Here's how the part is built. I have some questions about the finished solid (model axes, mm). Round coordinates to 2 decimals unless told otherwise and drop trailing zeros. Order: outer loops, then holes, each group sorted by start corner. A loop starts at its lowest first (then second) coordinate and runs counter-clockwise, first axis right, second up.
Autodesk Inventor part; units mm, degrees
ref_plane "YZ Plane" through (0, 0, 0) normal (1, 0, 0) x (0, 1, 0)
ref_plane "XZ Plane" through (0, 0, 0) normal (0, 1, 0) x (-1, 0, 0)
ref_plane "XY Plane" through (0, 0, 0) normal (0, 0, 1) x (1, 0, 0)
sketch "Sketch14" plane through (0, 0, 0) normal (0, 0, 1) x (1, 0, 0)
  circle A0 centre (0, 0) radius 65
  dimension "d67" = 130
extrude "Extrusion10" add sketch "Sketch14" along normal blind 6
sketch "Sketch15" plane through (0, 0, 6) normal (0, 0, 1) x (1, 0, 0)
  circle A0 centre (-37.7323, 38.6299) radius 2
  line L0 (-37.7323, 38.6299) -> (0, 0) construction
  circle A1 centre (0, 0) radius 65
  line L1 (0, 0) -> (-55.3564, 56.6733) construction
  line L2 (-55.3564, 56.6733) -> (-63.1164, 49.0935) construction
  dimension "d70" = 54
  dimension "d75" = 4
extrude "Extrusion11" cut sketch "Sketch15" against normal blind 6 contours A0
sketch "Sketch16" plane through (0, 0, 6) normal (0, 0, 1) x (1, 0, 0)
  circle A0 centre (-37.7323, 38.6299) radius 2.75
  circle A1 centre (-37.7323, 38.6299) radius 2
  point P0 (0, 0)
  dimension "d73" = 5.5
extrude "Extrusion12" add sketch "Sketch16" along normal blind 8
sketch "Sketch17" plane through (0, 0, 6) normal (0, 0, 1) x (1, 0, 0)
  circle A0 centre (-37.7323, 38.6299) radius 2.75
  circle A1 centre (-37.7323, 38.6299) radius 2 construction
  line L0 (-37.7323, 38.6299) -> (0, 0) construction
  line L1 (-37.7323, 38.6299) -> (-45.4185, 46.499) construction
  circle A2 centre (0, 0) radius 65 construction
  dimension "d79" = 130
ref_plane "Work Plane18" through (-45.4185, 46.499, 6) normal (-0.6987, 0.7154, 0) x (-0.7154, -0.6987, 0)
sketch "Sketch18" plane through (-45.4185, 46.499, 6) normal (-0.6987, 0.7154, 0) x (-0.7154, -0.6987, 0)
  line L0 (-2.7631, 8) -> (2.8739, 3.2761)
  line L1 (2.8739, 3.2761) -> (2.8739, 8)
  line L2 (2.8739, 8) -> (-2.7631, 8)
  point P0 (0, -6)
extrude "Extrusion13" cut sketch "Sketch18" against normal blind 15
pattern_circular "Circular Pattern2" count 10 over 360 about axis through (0, 0, 6) along (0, 0, 1) of "Extrusion12", "Extrusion13", "Extrusion11"
properties part number "inner bayonet connector 10"
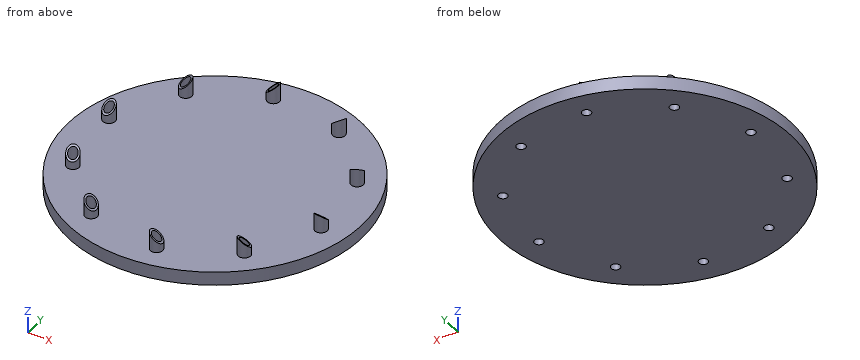
1. If we section it at B-B, the plane y = 33: Write out the boundary of the cut face in (x, z), and give its area (3 significant figures).
Evaluation:
outline: (-56, 0) - (56, 0) - (56, 6) - (-56, 6) - close
area: 672 mm2
2. I'm going to push flat-ended pins straight in: P1, Ø6, axis at y = -38, z = 3.5, coming from the +X side; P2, Ø1, axis at x = -14, z = 4.5, coming from the -Y side; P3, Ø4.5, axis at x = -7.82, y = 53.43, coming from the +Z side. Where does each tip first touch, or does it pass through?
Evaluation:
P1: stops at x = 54.77
P2: stops at y = -63.58
P3: stops at z = 13.57
3. I need wall thicknesses on probe 1 along X at (y, z) = (-45.5, 1); probe 2 along Y at (x, z) = (53.5, 3.25); probe 3 along Z at (x, y) = (-47, 11.5). Which ranges of each line are inside material? Lowest first, please.
Evaluation:
probe 1: x = -46.42 to 46.42
probe 2: y = -36.92 to -11.06, -7.09 to 36.92
probe 3: z = 0 to 6
4. If we section it at D-D, the plane z = 2.25: State how many separate pieces and enclosed holes the cut face has, and give its area (3 significant figures).
Evaluation:
separate pieces: 1
enclosed holes: 10
area: 13,100 mm2
5. If we section it at C-C, the plane x = 0: Write out the boundary of the cut face in (y, z), and give its area (3 significant figures).
Evaluation:
outline: (-65, 0) - (65, 0) - (65, 6) - (-65, 6) - close
area: 780 mm2
